```python
from build123d import *

# Parameters (mm, degrees)
BOSS_EXTRUDE1_DEPTH      = 8
BOSS_EXTRUDE1_DEPTH_BACK = 3
SKETCH1_R                = 6
SKETCH1_R_2              = 4
SKETCH3_R                = 2
FILLET1_R                = 0.5
SKETCH4_R                = 1
CUT_EXTRUDE2_DEPTH       = 12.66190379


with BuildPart() as part:
    # Sketch1 → Boss-Extrude1 (new, two sides: drawn at the far end of the back side and taken through both)
    with BuildSketch(Plane.XY.offset(-BOSS_EXTRUDE1_DEPTH_BACK)):
        Circle(SKETCH1_R)
        Circle(SKETCH1_R_2, mode=Mode.SUBTRACT)
    extrude(amount=BOSS_EXTRUDE1_DEPTH + BOSS_EXTRUDE1_DEPTH_BACK)

    # Sketch3 → Cut-Revolve1 (revolve, cut)
    with BuildSketch(Plane(origin=(0, 0, 0), x_dir=(1, 0, 0), z_dir=(0, 1, 0)), mode=Mode.PRIVATE) as cut_revolve1_sk:
        with Locations((-7, 0)):
            Circle(SKETCH3_R)
    revolve(cut_revolve1_sk.sketch.rotate(Axis((0, 0, -3.036308444), (0, 0, 1)), 180), axis=Axis((0, 0, -3.036308444), (0, 0, 1)), mode=Mode.SUBTRACT)

    # Fillet1
    fillet1_edges = [part.edges().sort_by_distance(p)[0] for p in [
        (-4, 0, -3),
        (-4, 0, 8),
    ]]
    fillet(fillet1_edges, radius=FILLET1_R)

    # Sketch4 → Cut-Extrude2 (cut, through all)
    with BuildSketch(Plane(origin=(0, 0, 0), x_dir=(1, 0, 0), z_dir=(0, 1, 0))):
        with Locations(Location((0, -6.101025888, 0), (0, 0, 90))):
            Circle(SKETCH4_R)
    extrude(amount=CUT_EXTRUDE2_DEPTH, mode=Mode.SUBTRACT)


solid = part.part
```
Build history of the part. All positions in model axes, mm. A direction names the side the tool comes from. Coordinates: 2 decimals unless noted, no trailing zeros. Order: outer loops, then holes, each group sorted by start corner. A loop starts at its lowest first (then second) coordinate and runs counter-clockwise, first axis right, second up. Notation, with made-up numbers: M 64.5,77.5 L 96.5,77.5 A28 cw 96.5,112.5 Z; hole C 72,31 d3. An arc over 180 degrees is marked long. One line per question, with ' | ' between items. Start each with the question number.
1. Cut at A-A (x = 0). Write the cut outline in (y, z), plus the area to 3 significant figures.
2. Wall check: line 1 along Y through (x, z) = (0, 0.5); line 2 along Y through (x, z) = (0, 2.75); line 3 along Y through (x, z) = (0, 6.5). Give the ranges that are in metal, low to high. Write a range as [from, to].
3. Mould opens along X. For faces 1 (the face through (-1.4, 4.5, 8)), 2 (the face through (-0.867, -3.905, 2.43)), 3 (the face through (-6, 0, -2)) say: +X half, -X half, draft (parallel to the pull), parting line (faces both ways), or undercut.
4. Cut at C-C (z = 2.5). Write the cut outline in (x, y), plus the area to 3 significant figures.
5. Cut at B-B (y = 0). Write the cut outline in (x, z), plus the area to 3 significant figures.
6. Tool access for faces 4 (the face through (-1.4, 4.5, -3)), 5 (the face through (0, 4.9, 7.1)): list every direction of +Z, -Z, +X, -X, +Y, -Y with a clear straight run to the whole face (end or side of a thin tool).
7. Flat gauge pins, fed straight in: P1, Ø4, axis at x = 0.5, y = -3, coming from the -Z side; P2, Ø1.5, axis at x = 2, z = -0.5, coming from the +Y side; P3, Ø1, axis at x = 2, z = 4, coming from the +Y side; P4, Ø1.5, axis at x = -3, z = 5.5, coming from the -Y side. Where does each tip first touch, or does it go through?
8. Cut at D-D (z = -1.5). Write the cut outline in (x, y), plus the area to 3 significant figures.
The answers:
1) outline: M -6,-3 L -4.5,-3 A0.5 ccw -4,-2.5 L -4,7.5 A0.5 ccw -4.5,8 L -6,8 L -6,1.73 A2 cw -6,-1.73 Z; M 4,-2.5 A0.5 ccw 4.5,-3 L 6,-3 L 6,-1.73 A2 cw 6,1.73 L 6,5.1 L 4,5.1 Z; M 4,7.1 L 6,7.1 L 6,8 L 4.5,8 A0.5 ccw 4,7.5 Z | area: 34.9 mm2
2) line 1: y = [-5.06, -4], [4, 5.06] | line 2: y = [-6, -4], [4, 6] | line 3: y = [-6, -4]
3) face 1: draft | face 2: undercut | face 3: parting line
4) outline: C 0,0 d12; hole C 0,0 d8 | area: 62.8 mm2
5) outline: M -6,-3 L -4.5,-3 A0.5 ccw -4,-2.5 L -4,7.5 A0.5 ccw -4.5,8 L -6,8 L -6,1.73 A2 cw -6,-1.73 Z; M 4,-2.5 A0.5 ccw 4.5,-3 L 6,-3 L 6,-1.73 A2 cw 6,1.73 L 6,8 L 4.5,8 A0.5 ccw 4,7.5 Z | area: 38.9 mm2
6) face 4: -Z, +X, -X, +Y, -Y | face 5: +Y
7) P1: stops at z = -3 | P2: stops at y = 5.12 | P3: stops at y = 5.81 | P4: stops at y = -5.56
8) outline: C 0,0 d11.35; hole C 0,0 d8 | area: 51.0 mm2
